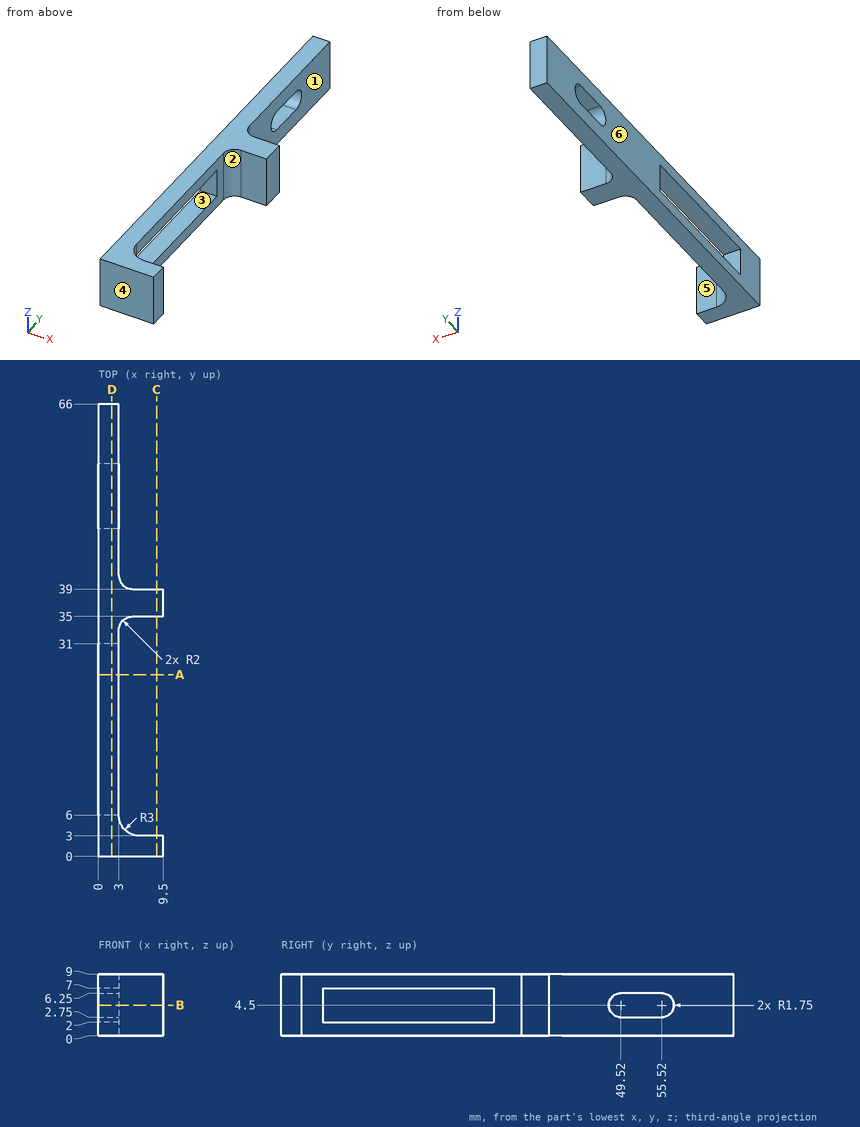
Design review of the part shown in the three views and the two pictorial views. Dimensions are in mm from the part's minimum x, y and z. A direction names the side the tool comes from. Coordinates: 2 decimals unless noted, no trailing zeros. Write each loop counter-clockwise with the first axis right and the second up, starting at its lowest first coordinate (ties: lowest second). Pieces come first, ordered by that corner, then holes. Notation, with made-up numbers: (11, -33) -> (50, -33) arc R23 ccw to (50, -11) -> close; hole circle Ø9 at (6.25, 31.5). An arc over 180 degrees is marked (long way). Answer in a Markdown table with one row per item.
1. For the marked faces 1, 2 and 3, list the 3-axis set-ups (+Z, -Z, +X, -X, +Y, -Y) from which the entire face can be reached by the end or side of a thin tool; tool diameter is ignored.
Answers below:
| item | result |
|---|---|
| face 1 | +Z, -Z, +X, +Y |
| face 2 | +Z, -Z, +X |
| face 3 | +X, -X |
2. Clearance check with flat-ended pins moving along their axes: pin 1 Ø5 at (x, z) = (7.5, 2.5) entering from +Y; pin 2 Ø1 at (x, z) = (4.5, 3.5) entering from +Y; pin 3 Ø4.5 at (y, z) = (20, 4) entering from +X. State where each tip first meets the part, or that it passes through.
Answers below:
| item | result |
|---|---|
| pin 1 | stops at y = 39 |
| pin 2 | stops at y = 39.27 |
| pin 3 | stops at x = 3 |
3. We need section D-D, the plane x = 2. State the section outline as (y, z) points.
Answers below:
| item | result |
|---|---|
| outline | (0, 0) -> (66, 0) -> (66, 9) -> (0, 9) -> close; hole (6, 2) -> (31, 2) -> (31, 7) -> (6, 7) -> close; hole (49.52, 2.75) -> (55.52, 2.75) arc R1.75 ccw to (55.52, 6.25) -> (49.52, 6.25) arc R1.75 ccw to start |
4. We need section A-A, the plane y = 26.5. State the section outline as (x, z) points.
Answers below:
| item | result |
|---|---|
| outline | (0, 0) -> (3, 0) -> (3, 2) -> (0, 2) -> close; (0, 7) -> (3, 7) -> (3, 9) -> (0, 9) -> close |
5. We need section C-C, the plane x = 8.5. State the section outline as (y, z) points, and give its area (3 significant figures).
Answers below:
| item | result |
|---|---|
| outline | (0, 0) -> (3, 0) -> (3, 9) -> (0, 9) -> close; (35, 0) -> (39, 0) -> (39, 9) -> (35, 9) -> close |
| area | 63.0 mm^2 |
6. Draft analysis for pull direction Y (two halves, no side actions). For the marked faces 4, 5 and 6, state which applies: +Y half, -Y half, draft (parallel to the pull), parting line (faces both ways), or undercut.
Answers below:
| item | result |
|---|---|
| face 4 | -Y half |
| face 5 | undercut |
| face 6 | draft |
7. We need section B-B, the plane z = 4.5. Give the number of separate pieces and of enclosed holes in the cut face, and give its area (3 significant figures).
Answers below:
| item | result |
|---|---|
| separate pieces | 3 |
| enclosed holes | 0 |
| area | 144 mm^2 |
8. Wall thickness on probe 1 along Z at (x, y) = (1.75, 18); probe 2 along Y at (x, z) = (8.75, 1.25); probe 3 along X at (y, z) = (12, 7.75): over which ranges is each line inside the solid? List them lowest first. Write a range as [from, to].
Answers below:
| item | result |
|---|---|
| probe 1 | z = [0, 2], [7, 9] |
| probe 2 | y = [0, 3], [35, 39] |
| probe 3 | x = [0, 3] |
